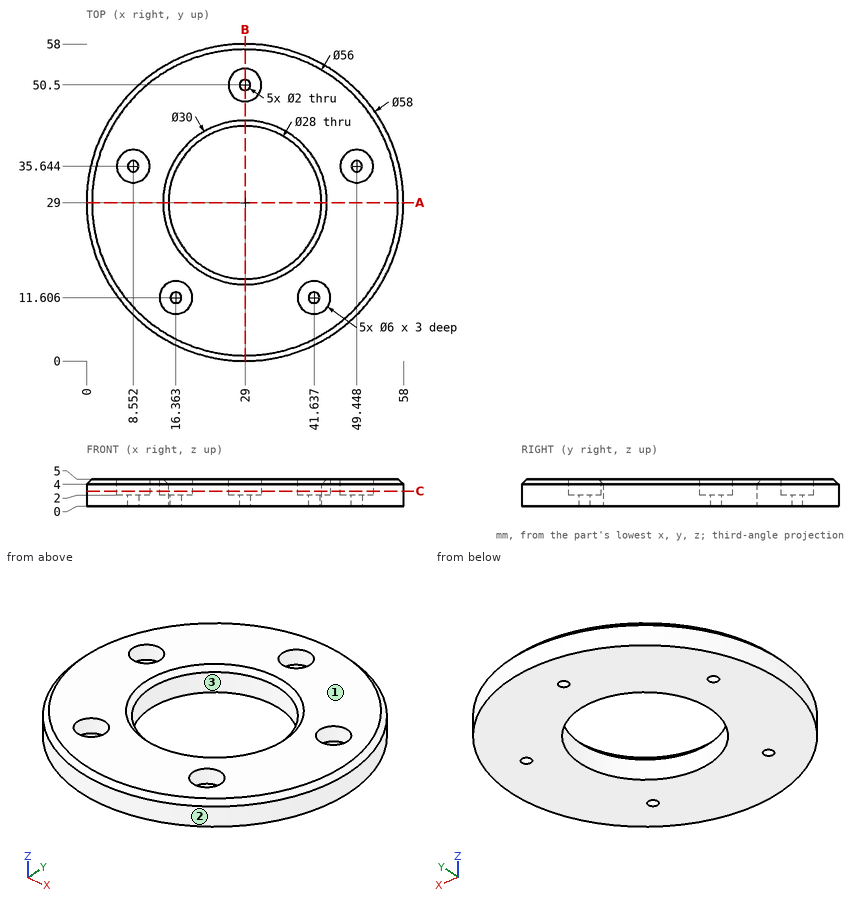
The drawing under review shows one solid part. Ordinate dimensions are in mm from its lowest x, y, z. Give positions to 0.01 mm unless a question says otherwise; leave off trailing zeros. Write each loop counter-clockwise with the first axis right and the second up, starting at its lowest first coordinate (ties: lowest second). Pieces come first, ordered by that corner, then holes. Notation, with made-up numbers: M 42,-38.75 L 87,-38.75 A22 ccw 87,-1.75 Z; hole C 79,33.25 d9. An arc over 180 degrees is marked long. Write each question's results on one line, items separated by ' | '. Start each with the question number.
1. We need section C-C (z = 2.8). Write out the cut boundary in (x, y), and give its area (4 significant figures).
2. Insertion check: pin 1 Ø2.5 at (x, y) = (41.64, 11.61) entering from +Z; pin 2 Ø3 at (y, z) = (38.5, 4.5) entering from -X; pin 3 Ø1.5 at (y, z) = (47.5, 4.5) entering from -X (1 decimal). Each pin has a flat end and moves straight along its axis. Give the tip position at first contact, or say it passes through.
3. Mouldability with a two-part tool opening along X and no side actions: class the marked faces 1, 2 and 3 as released by +X, released by -X, zero draft, split by the parting line, or undercut.
4. We need section B-B (x = 29). Write out the cut boundary in (y, z).
5. We need section A-A (y = 29). Write out the cut boundary in (x, z), and give its area (3 significant figures).
6. For probe 1 along Y at (x, z) = (41.5, 4.7) (1 decimal); probe 2 along Y at (x, z) = (39, 2.2) (1 decimal); probe 3 along Z at (x, y) = (7, 35), list the stretches that pass through material, from the lowest coordinate up. Write a range as [from, to].
Results found:
1) outline: C 29,29 d58; hole C 8.55,35.64 d6; hole C 16.36,11.61 d6; hole C 29,29 d28; hole C 29,50.5 d6; hole C 41.64,11.61 d6; hole C 49.45,35.64 d6 | area: 1,885 mm^2
2) pin 1: stops at z = 2 | pin 2: stops at x = 1.15 | pin 3: stops at x = 6.2
3) face 1: zero draft | face 2: split by the parting line | face 3: undercut
4) outline: M 0,0 L 15,0 L 15,4 L 14,5 L 1,5 L 0,4 Z; M 43,0 L 49.5,0 L 49.5,2 L 47.5,2 L 47.5,5 L 44,5 L 43,4 Z; M 51.5,0 L 58,0 L 58,4 L 57,5 L 53.5,5 L 53.5,2 L 51.5,2 Z
5) outline: M 0,0 L 15,0 L 15,4 L 14,5 L 1,5 L 0,4 Z; M 43,0 L 58,0 L 58,4 L 57,5 L 44,5 L 43,4 Z | area: 148 mm^2
6) probe 1: y = [3.6, 8.6], [14.6, 21.3], [36.7, 54.4] | probe 2: y = [1.8, 10.2], [13, 19.2], [38.8, 56.2] | probe 3: z = [0, 2]
